The model under review builds one solid part; all positions refer to its coordinate system, in mm. Face numbers are marked on the shaded views. A direction names the side the tool comes from. Round coordinates to 2 decimals unless told otherwise and drop trailing zeros. Loops run counter-clockwise (first coordinate to the right, second up) from the corner with the lowest first, then second, coordinate; pieces in that order, holes last. Notation, with made-up numbers: (-25.75, 82.25) - (-15.75, 82.25) arc R16 cw to (-15.75, 105.25) - close; hole circle Ø1 at (4.5, -17.75). An arc over 180 degrees is marked (long way). Answer as CSV lines item,"result".
from build123d import *

# Parameters (mm, degrees)
SKETCH1_R           = 5.715
SKETCH1_R_2         = 3.96875
BOSS_EXTRUDE1_DEPTH = 4.6
SKETCH2_R           = 9.525
SKETCH2_R_2         = 5.715
BOSS_EXTRUDE2_DEPTH = 3.175
CHAMFER2_SIZE       = 0.254


with BuildPart() as part:
    # Sketch1 → Boss-Extrude1 (new body, symmetric)
    with BuildSketch(Plane.XY):
        Circle(SKETCH1_R)
        Circle(SKETCH1_R_2, mode=Mode.SUBTRACT)
    extrude(amount=BOSS_EXTRUDE1_DEPTH, both=True)

    # Sketch2 → Boss-Extrude2 (add)
    with BuildSketch(Plane.XY.offset(4.6)):
        Circle(SKETCH2_R)
        Circle(SKETCH2_R_2, mode=Mode.SUBTRACT)
    extrude(amount=-BOSS_EXTRUDE2_DEPTH)

    # Chamfer2
    chamfer2_edges = [part.edges().sort_by_distance(p)[0] for p in [
        (-9.525, 0, 1.425),
        (-9.525, 0, 4.6),
        (-5.715, 0, -4.6),
    ]]
    chamfer(chamfer2_edges, length=CHAMFER2_SIZE)


solid = part.part
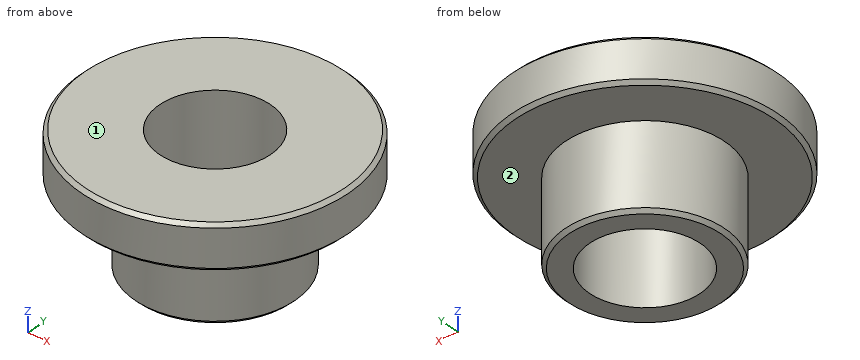
1. Wall thickness on probe 1 along Y at (x, z) = (0, 2) (3 decimals); probe 2 along Y at (x, z) = (0, -1.75) (3 decimals); probe 3 along Z at (x, y) = (6.25, 5.5) (3 decimals): over which ranges is each line inside the solid? List them lowest first.
Numbers:
probe 1,"y = -9.525 to -3.969, 3.969 to 9.525"
probe 2,"y = -5.715 to -3.969, 3.969 to 5.715"
probe 3,"z = 1.425 to 4.6"
2. Take a section at A-A (y = 0). State the section outline as (x, z) points (3 decimals), plus the area to 3 significant figures.
Numbers:
outline,"(-9.525, 1.679) - (-9.271, 1.425) - (-5.715, 1.425) - (-5.715, -4.346) - (-5.461, -4.6) - (-3.969, -4.6) - (-3.969, 4.6) - (-9.271, 4.6) - (-9.525, 4.346) - close; (3.969, -4.6) - (5.461, -4.6) - (5.715, -4.346) - (5.715, 1.425) - (9.271, 1.425) - (9.525, 1.679) - (9.525, 4.346) - (9.271, 4.6) - (3.969, 4.6) - close"
area,"56.1 mm²"
3. Take a section at C-C (z = -3.5). State the section outline as (x, y) points (1 decimal), plus the area to 3 significant figures.
Numbers:
outline,"circle Ø11.4 at (0, 0); hole circle Ø7.9 at (0, 0)"
area,"53.1 mm²"
4. Tool access review of the marked faces 1 and 2: name each direction out of +Z, -Z, +X, -X, +Y, -Y from which nothing blocks a thin tool from reaching the whole face with its end or side.
Numbers:
face 1,"+Z, +X, -X, +Y, -Y"
face 2,"-Z"
5. Clearance check with flat-ended pins moving along their axes: pin 1 (6.5 mm diameter, centred on x = 0, y = 0, fed in from -Z); pin 2 (1 mm diameter, centred on y = -6, z = 2, fed in from -X); pin 3 (1 mm diameter, centred on x = 4, z = 0.5, fed in from +Y); pin 4 (5 mm diameter, centred on y = -6.5, z = 3, fed in from -X). State where each tip first meets the part, or that it passes through.
Numbers:
pin 1,"passes through"
pin 2,"stops at x = -7.78"
pin 3,"stops at y = 4.52"
pin 4,"stops at x = -8.64"
